```python
from build123d import *

# Parameters (mm, degrees)
SKETCH_1_R          = 8
EXTRUDE_1_DEPTH     = 3
HOLE_WIZARD_M31_D   = 3.4
HOLE_WIZARD_M51_D   = 5.5
HOLE_WIZARD_M52_D   = 5.5
FILLET_1_R          = 10
FILLET_2_R          = 5
SKETCH_9_R          = 9
CUT_EXTRUDE_2_DEPTH = 1
CUT_EXTRUDE_3_DEPTH = 195.061830596
CUT_EXTRUDE_4_DEPTH = 195.061830596
CUT_EXTRUDE_6_DEPTH = 195.061830596
FILLET_6_R          = 4


with BuildPart() as part:
    # Эскиз1 → Бобышка-Вытянуть1 (new body)
    with BuildSketch(Plane.XY):
        with BuildLine():
            Line((-9.508526364, -3.096437692), (-1.398717752, -28))
            Line((-1.398717752, -28), (189.947361129, -28))
            ThreePointArc((189.947361129, -28), (191.995297124, 1.34383112), (189.536809823, 30.656120467))
            Line((189.536809823, 30.656120467), (125.388049295, 13.526041997))
            ThreePointArc((125.388049295, 13.526041997), (123.105499175, 12.698616461), (121.000225207, 11.489282104))
            Line((121.000225207, 11.489282104), (83.76563687, -14.436473614))
            Line((83.76563687, -14.436473614), (63.718090084, -22))
            Line((63.718090084, -22), (35.731449132, -22))
            Line((35.731449132, -22), (20.675178874, -13.02912429))
            Line((20.675178874, -13.02912429), (8.326583423, 5.537870395))
            ThreePointArc((8.326583423, 5.537870395), (-4.357415095, 9.00071851), (-9.508526364, -3.096437692))
        make_face()
        with Locations((129, 0)):
            Circle(SKETCH_1_R, mode=Mode.SUBTRACT)
    extrude(amount=EXTRUDE_1_DEPTH)

    # Отверстие с зазором M31 (through all)
    with Locations(Plane.XY.offset(3)):
        with Locations((9, -25), (40.5, -25), (72, -25)):
            Hole(HOLE_WIZARD_M31_D / 2)

    # Отверстие с зазором M51 (through all)
    with Locations(Plane.XY.offset(3)):
        with Locations((0, 0)):
            Hole(HOLE_WIZARD_M51_D / 2)

    # Отверстие с зазором M52 (through all)
    with Locations(Plane.XY.offset(3)):
        with Locations((183.228106674, 16.836297834), (183.914180714, 5.619086431), (183.914180714, -5.619086431), (183.228106674, -16.836297834)):
            Hole(HOLE_WIZARD_M52_D / 2)

    # Скругление1
    fillet_1_edges = [part.edges().sort_by_distance(p)[0] for p in [
        (35.731449132, -22, 1.5),
        (63.718090084, -22, 1.5),
        (83.76563687, -14.436473614, 1.5),
        (189.536809823, 30.656120467, 1.5),
        (189.947361129, -28, 1.5),
        (20.675178874, -13.02912429, 1.5),
    ]]
    fillet(fillet_1_edges, radius=FILLET_1_R)

    # Скругление2
    fillet_2_edges = [part.edges().sort_by_distance(p)[0] for p in [
        (-1.398717752, -28, 1.5),
    ]]
    fillet(fillet_2_edges, radius=FILLET_2_R)

    # Эскиз9 → Вырез-Вытянуть2 (cut)
    with BuildSketch(Plane(origin=(0, 0, 0), x_dir=(-1, 0, 0), z_dir=(0, 0, -1))):
        with Locations((-129, 0)):
            Circle(SKETCH_9_R)
    extrude(amount=-CUT_EXTRUDE_2_DEPTH, mode=Mode.SUBTRACT)

    # Эскиз10 → Вырез-Вытянуть3 (cut, through all)
    with BuildSketch(Plane.XY.offset(3)):
        with BuildLine():
            Line((6.5, -23.3), (11.5, -23.3))
            ThreePointArc((11.5, -23.3), (13.2, -25), (11.5, -26.7))
            Line((11.5, -26.7), (6.5, -26.7))
            ThreePointArc((6.5, -26.7), (4.8, -25), (6.5, -23.3))
        make_face()
        with BuildLine():
            Line((38, -23.3), (43, -23.3))
            ThreePointArc((43, -23.3), (44.7, -25), (43, -26.7))
            Line((43, -26.7), (38, -26.7))
            ThreePointArc((38, -26.7), (36.3, -25), (38, -23.3))
        make_face()
        with BuildLine():
            Line((69.5, -23.3), (74.5, -23.3))
            ThreePointArc((74.5, -23.3), (76.2, -25), (74.5, -26.7))
            Line((74.5, -26.7), (69.5, -26.7))
            ThreePointArc((69.5, -26.7), (67.8, -25), (69.5, -23.3))
        make_face()
    extrude(amount=-CUT_EXTRUDE_3_DEPTH, mode=Mode.SUBTRACT)

    # Эскиз12 → Вырез-Вытянуть4 (cut, through all)
    with BuildSketch(Plane(origin=(0, 0, 0), x_dir=(-1, 0, 0), z_dir=(0, 0, -1))):
        with BuildLine():
            Line((-178.522421187, -27.714873589), (-125.388049295, -13.526041997))
            ThreePointArc((-125.388049295, -13.526041997), (-115, 0), (-125.388049295, 13.526041997))
            Line((-125.388049295, 13.526041997), (17.708535377, 18.690586902))
            Line((17.708535377, 18.690586902), (9.18577518, -30.07854089))
            Line((9.18577518, -30.07854089), (-194.865610091, -30.07854089))
            Line((-194.865610091, -30.07854089), (-191.053066524, -19.0453609))
            ThreePointArc((-191.053066524, -19.0453609), (-186.79202351, -26.277041029), (-178.522421187, -27.714873589))
        make_face()
    extrude(amount=-CUT_EXTRUDE_4_DEPTH, mode=Mode.SUBTRACT)

    # Эскиз14 → Вырез-Вытянуть6 (cut, through all)
    with BuildSketch(Plane(origin=(0, 0, 0), x_dir=(-1, 0, 0), z_dir=(0, 0, -1))):
        with BuildLine():
            Line((-174.915688269, 19.506460401), (-146.526487717, 11.925499691))
            Line((-146.526487717, 11.925499691), (-174.915688269, -19.506460401))
            ThreePointArc((-174.915688269, -19.506460401), (-176, 0), (-174.915688269, 19.506460401))
        make_face()
        with BuildLine():
            Line((-139.389594338, 9.383833412), (-162.485080357, -16.187030888))
            Line((-162.485080357, -16.187030888), (-138.90792063, -9.891062066))
            ThreePointArc((-138.90792063, -9.891062066), (-142.995630653, -0.349746504), (-139.389594338, 9.383833412))
        make_face()
    extrude(amount=-CUT_EXTRUDE_6_DEPTH, mode=Mode.SUBTRACT)

    # Скругление6
    fillet_6_edges = [part.edges().sort_by_distance(p)[0] for p in [
        (174.915688269, -19.506460401, 1.5),
        (174.915688269, 19.506460401, 1.5),
        (146.526487717, 11.925499691, 1.5),
        (139.389594338, 9.383833412, 1.5),
        (138.90792063, -9.891062066, 1.5),
        (162.485080357, -16.187030888, 1.5),
    ]]
    fillet(fillet_6_edges, radius=FILLET_6_R)


solid = part.part
```
The model under review builds one solid part; all positions refer to its coordinate system, in mm. A direction names the side the tool comes from. Round coordinates to 2 decimals unless told otherwise and drop trailing zeros. Loops run counter-clockwise (first coordinate to the right, second up) from the corner with the lowest first, then second, coordinate; pieces in that order, holes last. Notation, with made-up numbers: M 75.25,55.5 L 91.25,55.5 A22 ccw 91.25,74.5 Z; hole C -12.75,-32.75 d3. An arc over 180 degrees is marked long. Write item = value, one per line.
Item 1: Take a section at C-C on z = 1.6. Write out the cut boundary in (x, y).
Return value:
outline = M 125.39,-13.53 L 178.52,-27.71 A10 ccw 180.07,-28 L 181.11,-28 A10 ccw 191.06,-18.99 A192 ccw 191.05,19.05 A10 ccw 178.52,27.71 L 125.39,13.53 A14 ccw Z; hole C 129,0 d16; hole M 141.73,-5.82 A4 ccw 144.34,-11.34 L 149.42,-12.7 A4 ccw 153.42,-6.15 L 149.42,-1.72 A4 ccw 142.57,-3.43 A14 cw Z; hole M 150.91,7.07 L 168.74,-12.67 A4 ccw 175.7,-10.22 A176 ccw 175.38,14.76 A4 ccw 170.36,18.29 L 152.85,13.61 A4 ccw Z; hole C 183.23,-16.84 d5.5; hole C 183.23,16.84 d5.5; hole C 183.91,-5.62 d5.5; hole C 183.91,5.62 d5.5
Item 2: Machinability: for faces 1 (the flat face through (162, -6, 0)), 2 (the flat face through (159.7, -2.66, 1.48)), which of the approach directions +Z, -Z, +X, -X, +Y, -Y give a long, thin tool a straight path to every point of the face, cutting with its end or side? Answer none if there is none.
Return value:
face_1 = -Z, +X, -X, +Y, -Y
face_2 = +Z, -Z
Item 3: Take a section at D-D on x = 159. Write out the cut boundary in (y, z).
Return value:
outline = M -22.5,0 L -1.88,0 L -1.88,3 L -22.5,3 Z; M 15.26,0 L 22.5,0 L 22.5,3 L 15.26,3 Z
Item 4: The part is to be moulded in two halves that separate along X. For faces 3 (the flat face through (162, -6, 3)), 4 (the cylindrical face through (192, 0, 1)), 5 (the cylindrical face through (142.2, -4.66, 1.48)), say which applies: released by +X, released by -X, zero draft, split by the parting line, or undercut.
Return value:
face_3 = zero draft
face_4 = released by +X
face_5 = undercut
Item 5: Insertion check: P1, Ø6.5, axis at x = 183.91, y = 5.62, coming from the +Z side. The pin has a flat end and moves straight along its axis. Give the tip position at first contact, or say it passes through.
Return value:
P1 = 3
Item 6: Take a section at A-A on x = 129. Write out the cut boundary in (y, z).
Return value:
outline = M -14.49,0 L -9,0 L -9,1 L -8,1 L -8,3 L -14.49,3 Z; M 8,1 L 9,1 L 9,0 L 14.49,0 L 14.49,3 L 8,3 Z
Item 7: For line 1 (X direction, y = -9.5, z = 2.1); line 2 (X direction, y = -11, z = 2.75); line 3 (X direction, y = 7, z = 1.45), list the stretches that pass through material, from the lowest coordinate up. Write a range as [from, to].
Return value:
line_1 = [118.72, 141.92], [154.4, 165.88], [175.74, 191.76]
line_2 = [120.34, 143.48], [153.82, 167.23], [175.58, 191.68]
line_3 = [116.88, 125.13], [132.87, 150.98], [175.86, 181.54], [186.29, 191.87]
Item 8: Take a section at B-B on y = 2. Write out the cut boundary in (x, z).
Return value:
outline = M 115.14,0 L 120.23,0 L 120.23,1 L 121.25,1 L 121.25,3 L 115.14,3 Z; M 136.75,1 L 137.77,1 L 137.77,0 L 155.49,0 L 155.49,3 L 136.75,3 Z; M 175.99,0 L 191.99,0 L 191.99,3 L 175.99,3 Z
